```python
from build123d import *
from OCP.BRepFilletAPI import BRepFilletAPI_MakeChamfer

# Parameters (mm, degrees)
SM_BASE_FLANGE_1_DEPTH = 57.5
CHAMFER_1_SIZE         = 40
CHAMFER_1_SIZE2        = 90
CHAMFER_2_SIZE         = 90
CHAMFER_2_SIZE2        = 40


# Sheet-metal steps are written as plain solids
with BuildPart() as part:
    # Sketch 1 → 基体-法兰1 (new, symmetric)
    with BuildSketch(Plane(origin=(0, 0, 0), x_dir=(0, 0, -1), z_dir=(1, 0, 0))):
        with BuildLine():
            Line((545, 0), (54.077004305, 0))
            ThreePointArc((54.077004305, 0), (47.981132154, 1.663639774), (43.575482564, 6.193276214))
            Line((43.575482564, 6.193276214), (1.498478259, 82.289986127))
            ThreePointArc((1.498478259, 82.289986127), (0.380657056, 85.09823204), (0, 88.096709913))
            Line((0, 88.096709913), (0, 765))
            Line((0, 765), (6, 765))
            Line((6, 765), (6, 88.096709913))
            ThreePointArc((6, 88.096709913), (6.190328528, 86.597470976), (6.74923913, 85.19334802))
            Line((6.74923913, 85.19334802), (48.826243434, 9.096638107))
            ThreePointArc((48.826243434, 9.096638107), (51.029068229, 6.831819887), (54.077004305, 6))
            Line((54.077004305, 6), (545, 6))
            Line((545, 6), (545, 0))
        make_face()
    extrude(amount=SM_BASE_FLANGE_1_DEPTH, both=True)

    # 倒角1: one chamfer whose edges measure the first distance from different faces: ONE call of the kernel's chamfer builder (chamfer() names one face for all edges)
    chamfer_1_edges_1 = [part.edges().sort_by_distance(p)[0] for p in [
        (-57.5, 765, -3),
    ]]
    chamfer_1_side_1 = [part.faces().sort_by_distance(p)[0] for p in [
        (0, 765, -3),
    ]]
    chamfer_1_edges_2 = [part.edges().sort_by_distance(p)[0] for p in [
        (-57.5, 3, -545),
    ]]
    chamfer_1_side_2 = [part.faces().sort_by_distance(p)[0] for p in [
        (0, 3, -545),
    ]]
    chamfer_1 = BRepFilletAPI_MakeChamfer(part.part.solid().wrapped)
    for e in chamfer_1_edges_1:
        chamfer_1.Add(CHAMFER_1_SIZE, CHAMFER_1_SIZE2, e.wrapped, chamfer_1_side_1[0].wrapped)  # the first distance lies on this face
    for e in chamfer_1_edges_2:
        chamfer_1.Add(CHAMFER_1_SIZE, CHAMFER_1_SIZE2, e.wrapped, chamfer_1_side_2[0].wrapped)  # the first distance lies on this face
    add(Compound.cast(chamfer_1.Shape()), mode=Mode.REPLACE)

    # 倒角2
    chamfer_2_edges = [part.edges().sort_by_distance(p)[0] for p in [
        (57.5, 765, -3),
        (57.5, 3, -545),
    ]]
    chamfer_2_side = [part.faces().sort_by_distance(p)[0] for p in [
        (57.5, 6.022757105, -50.551923163),
    ]]
    chamfer(chamfer_2_edges, length=CHAMFER_2_SIZE, length2=CHAMFER_2_SIZE2, reference=chamfer_2_side[0])


solid = part.part
```
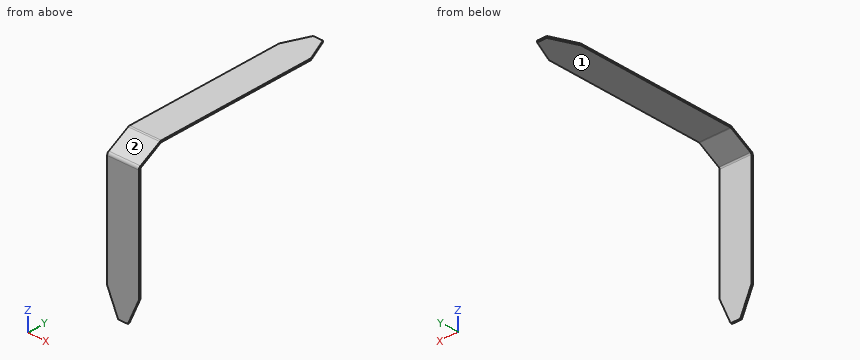
The model under review builds one solid part; all positions refer to its coordinate system, in mm. Face numbers are marked on the shaded views. A direction names the side the tool comes from. Round coordinates to 2 decimals unless told otherwise and drop trailing zeros. Write each loop counter-clockwise with the first axis right and the second up, starting at its lowest first coordinate (ties: lowest second). Pieces come first, ordered by that corner, then holes.
(1) Machinability: for the marked faces 1 and 2, which of the approach directions +Z, -Z, +X, -X, +Y, -Y give a long, thin tool a straight path to every point of the face, cutting with its end or side? Answer none if there is none.
(2) We need section B-B on y = 196. Give the boundary of the cut face in (x, z), and give its area (3 significant figures).
(3) Wall thickness on L1, parallel to Z at x = -53, y = 615.5; L2, parallel to Y at x = -50.5, z = -430: over which ranges is each line inside the solid? List them lowest first.
(4) We need section C-C on z = -396. Give the boundary of the cut face in (x, y), and give its area (3 significant figures).
(5) We need section D-D on x = -27. Give the boundary of the cut face in (y, z) (3 decimals), and give its area (3 significant figures).
(6) We need section A-A on x = 40.5. Give the boundary of the cut face in (y, z).
(7) Insertion check: pin 1 (2 mm diameter, centred on x = -35, y = 650.5, fed in from -Z); pin 2 (12 mm diameter, centred on x = 3, z = -439.5, fed in from +Y). Each pin has a flat end and moves straight along its axis. Give the tip position at first contact, or say it passes through.
Findings below:
1. face 1: -Z, +X, -X, +Y
1. face 2: +Z, +X, -X, -Y
2. outline: (-57.5, -6) - (57.5, -6) - (57.5, 0) - (-57.5, 0) - close
2. area: 690 mm2
3. L1: z = -6 to 0
3. L2: y = 0 to 6
4. outline: (-57.5, 0) - (57.5, 0) - (57.5, 6) - (-57.5, 6) - close
4. area: 690 mm2
5. outline: (0, -523.625) - (6, -523.625) - (6, -54.077) arc R6 cw to (9.097, -48.826) - (85.193, -6.749) arc R6 cw to (88.097, -6) - (743.625, -6) - (743.625, 0) - (88.097, 0) arc R12 ccw to (82.29, -1.498) - (6.193, -43.575) arc R12 ccw to (0, -54.077) - close
5. area: 7,360 mm2
6. outline: (0, -493.25) - (6, -493.25) - (6, -54.08) arc R6 cw to (9.1, -48.83) - (85.19, -6.75) arc R6 cw to (88.1, -6) - (713.25, -6) - (713.25, 0) - (88.1, 0) arc R12 ccw to (82.29, -1.5) - (6.19, -43.58) arc R12 ccw to (0, -54.08) - close
7. pin 1: stops at z = -6
7. pin 2: stops at y = 6
